```python
from build123d import *

# Parameters (mm, degrees)
SKETCH1_W                                   = 350
SKETCH1_H                                   = 109.2
BOSS_EXTRUDE1_DEPTH                         = 25.4
CBORE_FOR_0_BINDING_HEAD_MACHINE_SC_2_COUNT = 2
CBORE_FOR_0_BINDING_HEAD_MACHINE_SC_2_PITCH = 58.4
CBORE_FOR_0_BINDING_HEAD_MACHINE_SC_3_COUNT = 2
CBORE_FOR_0_BINDING_HEAD_MACHINE_SC_3_PITCH = 130
CBORE_FOR_0_BINDING_HEAD_MACHINE_SC_4_COUNT = 2
CBORE_FOR_0_BINDING_HEAD_MACHINE_SC_4_PITCH = 58.4


with BuildPart() as part:
    # Sketch1 → Boss-Extrude1 (new body)
    with BuildSketch(Plane(origin=(0, 0, 0), x_dir=(1, 0, 0), z_dir=(0, 1, 0))):
        Rectangle(SKETCH1_W, SKETCH1_H)
    extrude(amount=BOSS_EXTRUDE1_DEPTH)

    # Sketch3 → CBORE for #0 Binding Head Machine Screw1 (revolve, cut)
    with BuildSketch(Plane(origin=(-162.3, 12.7, 54.6), x_dir=(0, -1, 0), z_dir=(1, 0, 0))):
        Polygon((0, 0), (0, 30.53416509), (0.889, 30), (0.889, 0.8128), (1.98501, 0.8128), (1.98501, 0.87249), (2.8575, 0), align=None)
    cbore_for_0_binding_head_machine_screw1 = revolve(axis=Axis((-162.3, 12.7, 60.95), (0, 0, -1)), mode=Mode.SUBTRACT)

    # Mirror1: CBORE for #0 Binding Head Machine Screw1 across plane
    add(cbore_for_0_binding_head_machine_screw1.mirror(Plane.XY), mode=Mode.SUBTRACT)

    # Sketch5 → CBORE for #0 Binding Head Machine Screw2 (revolve, cut)
    with BuildSketch(Plane(origin=(175, 12.7, 29.1995), x_dir=(0, 0, -1), z_dir=(0, 1, 0))):
        Polygon((0, 0), (0, 30.53416509), (0.889, 30), (0.889, 0.8128), (1.98501, 0.8128), (1.98501, 0.635), (2.62001, 0), align=None)
    cbore_for_0_binding_head_machine_screw2 = revolve(axis=Axis((181.35, 12.7, 29.1995), (-1, 0, 0)), mode=Mode.SUBTRACT)

    # CBORE for _0 Binding Head Machine Sc 2: CBORE for #0 Binding Head Machine Screw2 ×2
    with Locations(*[(0, 0, -i * CBORE_FOR_0_BINDING_HEAD_MACHINE_SC_2_PITCH) for i in range(1, CBORE_FOR_0_BINDING_HEAD_MACHINE_SC_2_COUNT)]):
        add(cbore_for_0_binding_head_machine_screw2, mode=Mode.SUBTRACT)

    # Sketch9 → CBORE for #0 Binding Head Machine Screw4 (revolve, cut)
    with BuildSketch(Plane(origin=(-65, 0, 0), x_dir=(0, 0, -1), z_dir=(1, 0, 0))):
        Polygon((0, 0), (0, 30.53416509), (0.889, 30), (0.889, 0.8128), (1.98501, 0.8128), (1.98501, 0.87249), (2.8575, 0), align=None)
    cbore_for_0_binding_head_machine_screw4 = revolve(axis=Axis((-65, -6.35, 0), (0, 1, 0)), mode=Mode.SUBTRACT)

    # CBORE for _0 Binding Head Machine Sc 3: CBORE for #0 Binding Head Machine Screw4 ×2
    with Locations(*[(i * CBORE_FOR_0_BINDING_HEAD_MACHINE_SC_3_PITCH, 0, 0) for i in range(1, CBORE_FOR_0_BINDING_HEAD_MACHINE_SC_3_COUNT)]):
        add(cbore_for_0_binding_head_machine_screw4, mode=Mode.SUBTRACT)

    # Sketch13 → CBORE for #0 Binding Head Machine Screw6 (revolve, cut)
    with BuildSketch(Plane(origin=(-162.3, 0, -29.2), x_dir=(0, 0, -1), z_dir=(1, 0, 0))):
        Polygon((0, 0), (0, 25.4), (0.889, 25.4), (0.889, 0.8128), (1.98501, 0.8128), (1.98501, 0.87249), (2.8575, 0), align=None)
    cbore_for_0_binding_head_machine_screw6 = revolve(axis=Axis((-162.3, -6.35, -29.2), (0, 1, 0)), mode=Mode.SUBTRACT)

    # CBORE for _0 Binding Head Machine Sc 4: CBORE for #0 Binding Head Machine Screw6 ×2
    with Locations(*[(0, 0, i * CBORE_FOR_0_BINDING_HEAD_MACHINE_SC_4_PITCH) for i in range(1, CBORE_FOR_0_BINDING_HEAD_MACHINE_SC_4_COUNT)]):
        add(cbore_for_0_binding_head_machine_screw6, mode=Mode.SUBTRACT)


solid = part.part
```
Design review of the part built by this model. Coordinates are the model's own, in mm. Coordinates: 2 decimals unless noted, no trailing zeros. One line per question, with ' | ' between items.
(1) Wall thickness on probe 1 along Z at (x, y) = (-65, 14.25); probe 2 along Z at (x, y) = (-162.3, 3); probe 3 along X at (y, z) = (12.7, -27.8): over which ranges is each line inside the solid? List them lowest first.
Filled in:
probe 1: z = -54.6 to -0.89, 0.89 to 54.6 | probe 2: z = -54.6 to -30.09, -28.31 to 28.31, 30.09 to 54.6 | probe 3: x = -175 to -163.19, -161.41 to 174.19
(2) For pin 1 Ø3 at (x, y) = (-162.3, 12.7) entering from +Z; pin 2 Ø2 at (x, z) = (65, 0) entering from +Y; pin 3 Ø1.2 at (x, z) = (-162, 29.5) entering from -Y; pin 4 Ø1.6 at (x, y) = (-162.3, 12.7) entering from -Z, all flat-tipped, find the tip position at first contact; note any pin that passes through.
Filled in:
pin 1: stops at z = 53.79 | pin 2: stops at y = 25.4 | pin 3: stops at y = 0.81 | pin 4: stops at z = -24.55
(3) Draft analysis for pull direction Z (two halves, no side actions). For faces 1 (the face through (-2, 13, -54.6)), 2 (the face through (-2, 13, 54.6)), 3 (the face through (-175, 13, 1)), state which applies: released by +Z, released by -Z, zero draft, split by the parting line, or undercut.
Filled in:
face 1: released by -Z | face 2: released by +Z | face 3: zero draft
